```python
from build123d import *

# Parameters (mm, degrees)
F1_DEPTH       = 165.1
F3_D           = 20.6375
F3_CBORE_D     = 30.1752
F3_CBORE_DEPTH = 28.448
F4_R           = 1.524


# Not quite as in the source:
# - a length typed as a fraction of an inch, garbled in the dataset ("3 / 203.2 mm" for 3/8 in), is restored


with BuildPart() as f1:
    # F0 (on Top) → F1 (new body, symmetric)
    with BuildSketch(Plane.XY):
        Polygon((95.25, 44.45), (-95.25, 44.45), (-95.25, 31.75), (-57.15, 31.75), (-57.15, -31.75), (-95.25, -31.75), (-95.25, -44.45), (95.25, -44.45), align=None)
    extrude(amount=F1_DEPTH, both=True)

    # F3 (through all)
    with Locations(Plane.YZ.offset(95.25)):
        with Locations((0, 107.95), (0, -107.95)):
            CounterBoreHole(F3_D / 2, F3_CBORE_D / 2, F3_CBORE_DEPTH)

    # F4
    f4_edges = [f1.edges().sort_by_distance(p)[0] for p in [
        (-57.15, 31.75, 0),
        (-57.15, -31.75, 0),
    ]]
    fillet(f4_edges, radius=F4_R)


solid = f1.part
```
The model under review builds one solid part; all positions refer to its coordinate system, in mm. A direction names the side the tool comes from. Round coordinates to 2 decimals unless told otherwise and drop trailing zeros. Write each loop counter-clockwise with the first axis right and the second up, starting at its lowest first coordinate (ties: lowest second). Pieces come first, ordered by that corner, then holes.
(1) Machinability: for faces 4 (the cylindrical face through (81.23, -1.96, -92.99)), 5 (the flat face through (95.25, -1, 2)), 6 (the flat face through (-57.15, 0, 2)), which of the approach directions +Z, -Z, +X, -X, +Y, -Y give a long, thin tool a straight path to every point of the face, cutting with its end or side? Answer none if there is none.
(2) Insertion check: pin 1 (18.5 mm diameter, centred on y = 0, z = -107.95, fed in from -X); pin 2 (23.5 mm diameter, centred on y = 0, z = 107.95, fed in from +X); pin 3 (8 mm diameter, centred on y = 15, z = -26.5, fed in from -X); pin 4 (5 mm diameter, centred on y = -24, z = -16, fed in from -X). Each pin has a flat end and moves straight along its axis. Give the tip position at first contact, or say it passes through.
(3) We need section D-D on y = 18.5. Give the boundary of the cut face in (x, z), and give its area (3 significant figures).
(4) Mouldability with a two-part tool opening along Z and no side actions: class faces 1 (the flat face through (1, 44.45, 2)), 2 (the flat face through (66.802, 3, -118)), 3 (the flat face through (20, 1, 165.1)) as +Z half, -Z half, draft (parallel to the pull), parting line (faces both ways), or undercut.
(5) Wall thickness on L1, parallel to Z at x = 21.5, y = 0; L2, parallel to Z at x = 89, y = 0; L3, parallel to Y at x = 74, z = -107: over which ranges is each line inside the solid? List them lowest first.
(6) We need section C-C on x = 37.5. Give the boundary of the cut face in (y, z), and give its area (3 significant figures).
(7) We need section A-A on y = 0. Give the boundary of the cut face in (x, z).
(8) We need section B-B on z = 107.95. Give the boundary of the cut face in (x, y).
Findings below:
1. face 4: +X
1. face 5: +Z, -Z, +X, +Y, -Y
1. face 6: +Z, -Z, -X
2. pin 1: passes through
2. pin 2: stops at x = 66.8
2. pin 3: stops at x = -57.15
2. pin 4: stops at x = -57.15
3. outline: (-57.15, -165.1) - (95.25, -165.1) - (95.25, 165.1) - (-57.15, 165.1) - close
3. area: 50,300 mm2
4. face 1: draft
4. face 2: undercut
4. face 3: +Z half
5. L1: z = -165.1 to -118.27, -97.63 to 97.63, 118.27 to 165.1
5. L2: z = -165.1 to -123.04, -92.86 to 92.86, 123.04 to 165.1
5. L3: y = -44.45 to -15.06, 15.06 to 44.45
6. outline: (-44.45, -165.1) - (44.45, -165.1) - (44.45, 165.1) - (-44.45, 165.1) - close; hole circle Ø20.64 at (0, -107.95); hole circle Ø20.64 at (0, 107.95)
6. area: 28,700 mm2
7. outline: (-57.15, -165.1) - (95.25, -165.1) - (95.25, -123.04) - (66.8, -123.04) - (66.8, -118.27) - (-57.15, -118.27) - close; (-57.15, -97.63) - (66.8, -97.63) - (66.8, -92.86) - (95.25, -92.86) - (95.25, 92.86) - (66.8, 92.86) - (66.8, 97.63) - (-57.15, 97.63) - close; (-57.15, 118.27) - (66.8, 118.27) - (66.8, 123.04) - (95.25, 123.04) - (95.25, 165.1) - (-57.15, 165.1) - close
8. outline: (-95.25, -44.45) - (95.25, -44.45) - (95.25, -15.09) - (66.8, -15.09) - (66.8, -10.32) - (-57.15, -10.32) - (-57.15, -30.23) arc R1.52 cw to (-58.67, -31.75) - (-95.25, -31.75) - close; (-95.25, 31.75) - (-58.67, 31.75) arc R1.52 cw to (-57.15, 30.23) - (-57.15, 10.32) - (66.8, 10.32) - (66.8, 15.09) - (95.25, 15.09) - (95.25, 44.45) - (-95.25, 44.45) - close
